Read the model definition and answer for the solid it produces. Units are mm, in the model's axes. Coordinates: 2 decimals unless noted, no trailing zeros. Order: outer loops, then holes, each group sorted by start corner. A loop starts at its lowest first (then second) coordinate and runs counter-clockwise, first axis right, second up. Notation, with made-up numbers: M 83.25,50.25 L 135.25,50.25 A28 ccw 135.25,78.25 Z; hole C 25,-31.5 d4. An arc over 180 degrees is marked long. Use a Markdown table: item, result. Add a question column.
1) Find section C-C on y = -4.25. Write down the section's boundary in (x, z), plus the area to 3 significant figures.
2) This flat-tipped pin is pushed along its axis until it touches: pin 1 Ø12 at (x, z) = (9.5, 7) entering from +Y. Where does it stop, or does it pass through?
3) Find section B-B on x = -3.75. Write down the section's boundary in (y, z), plus the area to 3 significant figures.
4) Find section A-A on z = 2. Write down the section's boundary in (x, y).
5) The mould has two halves that part along Z. Classify faces 1 (the face through (0, -6, 12.7)), 2 (the face through (3, 0, 0)), 3 (the face through (-4.66, -6.44, 1.63)): released by +Z, released by -Z, zero draft, split by the parting line, or undercut.
6) Find the intervals of material crossed by probe 1 along Z at (x, y) = (-1.25, -1.25); probe 2 along X at (y, z) = (-3.25, 1.5); probe 3 along Z at (x, y) = (2, -8.5), in increasing order. Write a range as [from, to].
Autodesk Inventor part; units mm, degrees
ref_plane "YZ Plane" through (0, 0, 0) normal (1, 0, 0) x (0, 1, 0)
ref_plane "XZ Plane" through (0, 0, 0) normal (0, 1, 0) x (-1, 0, 0)
ref_plane "XY Plane" through (0, 0, 0) normal (0, 0, 1) x (1, 0, 0)
sketch "Sketch1" plane through (0, 0, 0) normal (0, 1, 0) x (-1, 0, 0)
  line L0 (-12.7, 12.7) -> (-12.7, -12.7)
  line L1 (-12.7, -12.7) -> (12.7, -12.7)
  line L2 (12.7, -12.7) -> (12.7, 12.7)
  line L3 (12.7, 12.7) -> (-12.7, 12.7)
  line L4 (-12.7, 12.7) -> (12.7, -12.7) construction
  line L5 (-12.7, -12.7) -> (12.7, 12.7) construction
  point P0 (0, 0)
  dimension "d0" = 25.4
extrude "Extrusion1" add sketch "Sketch1" against normal blind 12.7
sketch "Sketch3" plane through (0, 0, 0) normal (0, 1, 0) x (1, 0, 0)
  point P0 (0, 0)
  point P1 (-1.3731, 0.4703)
hole "Hole2" at (-1.3731, 0, -0.4703) direction (0, -1, 0) diameter 7.7978 end through all
thread "Thread3"
properties part number "_3DPrint"
Check result:
| question | item | result |
|---|---|---|
| 1 | outline | M -12.7,-12.7 L 12.7,-12.7 L 12.7,12.7 L -12.7,12.7 Z; hole C -1.37,-0.47 d7.8 |
| 1 | area | 597 mm2 |
| 2 | pin 1 | stops at y = 0 |
| 3 | outline | M -12.7,-12.7 L 0,-12.7 L 0,-3.56 L -12.7,-3.56 Z; M -12.7,2.62 L 0,2.62 L 0,12.7 L -12.7,12.7 Z |
| 3 | area | 244 mm2 |
| 4 | outline | M -12.7,-12.7 L -4.39,-12.7 L -4.39,0 L -12.7,0 Z; M 1.64,-12.7 L 12.7,-12.7 L 12.7,0 L 1.64,0 Z |
| 5 | face 1 | released by +Z |
| 5 | face 2 | zero draft |
| 5 | face 3 | undercut |
| 6 | probe 1 | z = [-12.7, -4.37], [3.43, 12.7] |
| 6 | probe 2 | x = [-12.7, -4.74], [1.99, 12.7] |
| 6 | probe 3 | z = [-12.7, -2.43], [1.49, 12.7] |
